Geometry check sheet. Reference: the model listing, model coordinates, mm. Face numbers are marked on the shaded views. Round coordinates to 2 decimals unless told otherwise and drop trailing zeros. Order: outer loops, then holes, each group sorted by start corner. A loop starts at its lowest first (then second) coordinate and runs counter-clockwise, first axis right, second up. Notation, with made-up numbers: (3, -13.5) - (26, -13.5) arc R33 ccw to (26, 16.5) - close; hole circle Ø5 at (-7, -23.75). An arc over 180 degrees is marked (long way). Use a Markdown table: item, result. Add a question column.
(1) Section check B-B on x = 3.75. Record the boundary of the cut face in (y, z).
(2) Section check D-D on y = -3.75. Record the boundary of the cut face in (x, z), then the cut area to 3 significant figures.
(3) Thickness scan on line 1 along X through (y, z) = (1.5, 5.25). Record the ranges inside material, lowest first. Write a range as [from, to].
(4) Section check C-C on z = 3. Record the boundary of the cut face in (x, y).
(5) Mould release check, pull along Z, two halves, no side actions. Record for the marked faces 1, 2 and 3: released by +Z, released by -Z, zero draft, split by the parting line, or undercut.
(6) Section check A-A on y = 3.25. Record the boundary of the cut face in (x, z), then the cut area to 3 significant figures.
(7) Gauge pin test, flat ends, axial feed: P1, Ø2.5, axis at x = 4, z = 4.5, coming from the +Y side; P2, Ø0.7, axis at x = 3, z = 4.5, coming from the -Y side; P3, Ø1.5, axis at y = -2, z = 5, coming from the +X side. Record the tip position at first contact, or that the pin passes through.
```python
from build123d import *

# Parameters (mm, degrees)
SKETCH1_W                  = 4.7
SKETCH1_H                  = 9.2
BOSS_EXTRUDE1_DEPTH        = 8
BOSS_EXTRUDE2_DEPTH        = 0.5
FILLET1_R                  = 0.2
FILLET2_R                  = 0.2
LPATTERN2_COUNT            = 2
LPATTERN2_PITCH            = 3
FILLET1_OF_LPATTERN2_R     = 0.2
FILLET2_OF_LPATTERN2_R     = 0.2
LPATTERN2_COL_COUNT        = 2
LPATTERN2_COL_PITCH        = 3
FILLET1_OF_LPATTERN2_COL_R = 0.2
FILLET2_OF_LPATTERN2_COL_R = 0.2


with BuildPart() as part:
    # Sketch1 → Boss-Extrude1 (new body)
    with BuildSketch(Plane.XY):
        Rectangle(SKETCH1_W, SKETCH1_H)
    extrude(amount=BOSS_EXTRUDE1_DEPTH)

    # Sketch2 → Boss-Extrude2 (add, symmetric)
    with BuildSketch(Plane(origin=(0, 0, 0), x_dir=(1, 0, 0), z_dir=(0, 1, 0))):
        Polygon((2.35, -8), (4.65, -7.5), (2.35, -2.5), (2.35, -2.739288485), (4.507138989, -7.428721069), (2.35, -7.897664328), align=None)
    boss_extrude2 = extrude(amount=BOSS_EXTRUDE2_DEPTH, both=True)

    # Fillet1
    fillet1_edges = [part.edges().sort_by_distance(p)[0] for p in [
        (4.507138989, 0, 7.428721069),
    ]]
    fillet(fillet1_edges, radius=FILLET1_R)

    # Fillet2
    fillet2_edges = [part.edges().sort_by_distance(p)[0] for p in [
        (4.65, 0, 7.5),
    ]]
    fillet(fillet2_edges, radius=FILLET2_R)

    # LPattern2: Boss-Extrude2 ×2
    with Locations(*[(0, -i * LPATTERN2_PITCH, 0) for i in range(1, LPATTERN2_COUNT)]):
        add(boss_extrude2)

    # Fillet1 of LPattern2
    fillet1_of_lpattern2_edges = [part.edges().sort_by_distance(p)[0] for p in [
        (4.507138989, -3, 7.428721069),
    ]]
    fillet(fillet1_of_lpattern2_edges, radius=FILLET1_OF_LPATTERN2_R)

    # Fillet2 of LPattern2
    fillet2_of_lpattern2_edges = [part.edges().sort_by_distance(p)[0] for p in [
        (4.65, -3, 7.5),
    ]]
    fillet(fillet2_of_lpattern2_edges, radius=FILLET2_OF_LPATTERN2_R)

    # LPattern2 col: Boss-Extrude2 ×2
    with Locations(*[(0, i * LPATTERN2_COL_PITCH, 0) for i in range(1, LPATTERN2_COL_COUNT)]):
        add(boss_extrude2)

    # Fillet1 of LPattern2 col
    fillet1_of_lpattern2_col_edges = [part.edges().sort_by_distance(p)[0] for p in [
        (4.507138989, 3, 7.428721069),
    ]]
    fillet(fillet1_of_lpattern2_col_edges, radius=FILLET1_OF_LPATTERN2_COL_R)

    # Fillet2 of LPattern2 col
    fillet2_of_lpattern2_col_edges = [part.edges().sort_by_distance(p)[0] for p in [
        (4.65, 3, 7.5),
    ]]
    fillet(fillet2_of_lpattern2_col_edges, radius=FILLET2_OF_LPATTERN2_COL_R)


solid = part.part
```
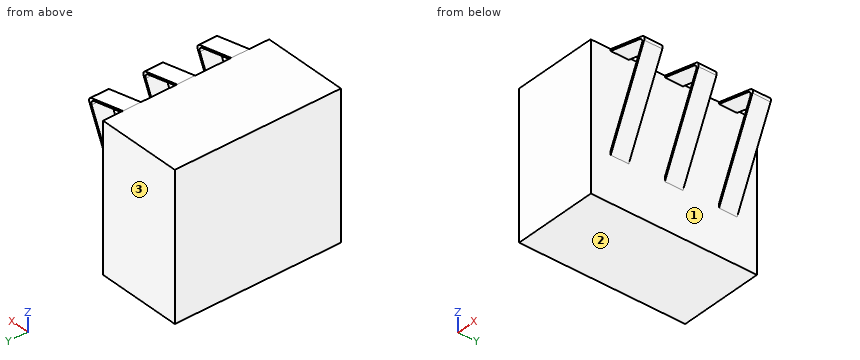
Check sheet entries:
| question | item | result |
|---|---|---|
| 1 | outline | (-3.5, 5.54) - (-2.5, 5.54) - (-2.5, 5.78) - (-3.5, 5.78) - close; (-3.5, 7.59) - (-2.5, 7.59) - (-2.5, 7.7) - (-3.5, 7.7) - close; (-0.5, 5.54) - (0.5, 5.54) - (0.5, 5.78) - (-0.5, 5.78) - close; (-0.5, 7.59) - (0.5, 7.59) - (0.5, 7.7) - (-0.5, 7.7) - close; (2.5, 5.54) - (3.5, 5.54) - (3.5, 5.78) - (2.5, 5.78) - close; (2.5, 7.59) - (3.5, 7.59) - (3.5, 7.7) - (2.5, 7.7) - close |
| 2 | outline | (-2.35, 0) - (2.35, 0) - (2.35, 8) - (-2.35, 8) - close |
| 2 | area | 37.6 mm2 |
| 3 | line 1 | x = [-2.35, 2.35] |
| 4 | outline | (-2.35, -4.6) - (2.35, -4.6) - (2.35, 4.6) - (-2.35, 4.6) - close; (2.47, -3.5) - (2.58, -3.5) - (2.58, -2.5) - (2.47, -2.5) - close; (2.47, -0.5) - (2.58, -0.5) - (2.58, 0.5) - (2.47, 0.5) - close; (2.47, 2.5) - (2.58, 2.5) - (2.58, 3.5) - (2.47, 3.5) - close |
| 5 | face 1 | undercut |
| 5 | face 2 | released by -Z |
| 5 | face 3 | zero draft |
| 6 | outline | (-2.35, 0) - (2.35, 0) - (2.35, 2.5) - (4.55, 7.27) arc R0.2 ccw to (4.41, 7.55) - (2.35, 8) - (-2.35, 8) - close; hole (2.35, 2.74) - (4.4, 7.2) arc R0.2 ccw to (4.26, 7.48) - (2.35, 7.9) - close |
| 6 | area | 38.4 mm2 |
| 7 | P1 | stops at y = 3.5 |
| 7 | P2 | stops at y = -3.5 |
| 7 | P3 | stops at x = 3.76 |
